from build123d import *

# Parameters (mm, degrees)
SKETCH1_R           = 9.175
SKETCH1_R_2         = 5.6
BOSS_EXTRUDE1_DEPTH = 1.25
CHAMFER1_SIZE       = 0.5
CUT_EXTRUDE1_REACH  = 4.5
CHAMFER2_SIZE       = 0.5


with BuildPart() as part:
    # Sketch1 → Boss-Extrude1 (new body, symmetric)
    with BuildSketch(Plane(origin=(0, 0, 0), x_dir=(1, 0, 0), z_dir=(0, 1, 0))):
        Circle(SKETCH1_R)
        Circle(SKETCH1_R_2, mode=Mode.SUBTRACT)
    extrude(amount=BOSS_EXTRUDE1_DEPTH, both=True)

    # Chamfer1
    chamfer1_edges = [part.edges().sort_by_distance(p)[0] for p in [
        (-9.175, -1.25, 0),
        (-9.175, 1.25, 0),
    ]]
    chamfer(chamfer1_edges, length=CHAMFER1_SIZE)

    # Sketch2 → Cut-Extrude1 (cut, up to next)
    with BuildSketch(Plane(origin=(0, 1.25, 0), x_dir=(1, 0, 0), z_dir=(0, 1, 0)), mode=Mode.PRIVATE) as cut_extrude1_sk1:
        with BuildLine():
            ThreePointArc((-8, 3.354940387), (-8.675, 0), (-8, -3.354940387))
            Line((-8, -3.354940387), (-8, 3.354940387))
        make_face()
    cut_extrude1_tool1 = extrude(cut_extrude1_sk1.sketch, amount=-CUT_EXTRUDE1_REACH, mode=Mode.PRIVATE) & part.part
    add(cut_extrude1_tool1.solids().sort_by_distance((-8.270921, 1.25, 0))[0], mode=Mode.SUBTRACT)
    # Sketch2 → Cut-Extrude1 (cut, up to next)
    with BuildSketch(Plane(origin=(0, 1.25, 0), x_dir=(1, 0, 0), z_dir=(0, 1, 0)), mode=Mode.PRIVATE) as cut_extrude1_sk2:
        with BuildLine():
            ThreePointArc((-8, 4.492285053), (-9.175, 0), (-8, -4.492285053))
            Line((-8, -4.492285053), (-8, -3.354940387))
            ThreePointArc((-8, -3.354940387), (-8.675, 0), (-8, 3.354940387))
            Line((-8, 3.354940387), (-8, 4.492285053))
        make_face()
    cut_extrude1_tool2 = extrude(cut_extrude1_sk2.sketch, amount=-CUT_EXTRUDE1_REACH, mode=Mode.PRIVATE) & part.part
    add(cut_extrude1_tool2.solids().sort_by_distance((-9.084389, 1.25, 0))[0], mode=Mode.SUBTRACT)
    # Sketch2 → Cut-Extrude1 (cut, up to next)
    with BuildSketch(Plane(origin=(0, 1.25, 0), x_dir=(1, 0, 0), z_dir=(0, 1, 0)), mode=Mode.PRIVATE) as cut_extrude1_sk3:
        with BuildLine():
            ThreePointArc((-0.109567023, 9.174345757), (-4.5875, 7.94578308), (-7.890432977, 4.682060704))
            Line((-7.890432977, 4.682060704), (-6.905463603, 5.250733037))
            ThreePointArc((-6.905463603, 5.250733037), (-4.3375, 7.512770378), (-1.094536397, 8.605673424))
            Line((-1.094536397, 8.605673424), (-0.109567023, 9.174345757))
        make_face()
    cut_extrude1_tool3 = extrude(cut_extrude1_sk3.sketch, amount=-CUT_EXTRUDE1_REACH, mode=Mode.PRIVATE) & part.part
    add(cut_extrude1_tool3.solids().sort_by_distance((-4.382423, 1.25, -7.590579))[0], mode=Mode.SUBTRACT)
    # Sketch2 → Cut-Extrude1 (cut, up to next)
    with BuildSketch(Plane(origin=(0, 1.25, 0), x_dir=(1, 0, 0), z_dir=(0, 1, 0)), mode=Mode.PRIVATE) as cut_extrude1_sk4:
        with BuildLine():
            ThreePointArc((-1.094536397, 8.605673424), (-4.3375, 7.512770378), (-6.905463603, 5.250733037))
            Line((-6.905463603, 5.250733037), (-1.094536397, 8.605673424))
        make_face()
    cut_extrude1_tool4 = extrude(cut_extrude1_sk4.sketch, amount=-CUT_EXTRUDE1_REACH, mode=Mode.PRIVATE) & part.part
    add(cut_extrude1_tool4.solids().sort_by_distance((-4.135461, 1.25, -7.162828))[0], mode=Mode.SUBTRACT)
    # Sketch2 → Cut-Extrude1 (cut, up to next)
    with BuildSketch(Plane(origin=(0, 1.25, 0), x_dir=(1, 0, 0), z_dir=(0, 1, 0)), mode=Mode.PRIVATE) as cut_extrude1_sk5:
        with BuildLine():
            ThreePointArc((1.094536397, 8.605673424), (4.3375, 7.512770378), (6.905463603, 5.250733037))
            Line((6.905463603, 5.250733037), (7.890432977, 4.682060704))
            ThreePointArc((7.890432977, 4.682060704), (4.5875, 7.94578308), (0.109567023, 9.174345757))
            Line((0.109567023, 9.174345757), (1.094536397, 8.605673424))
        make_face()
    cut_extrude1_tool5 = extrude(cut_extrude1_sk5.sketch, amount=-CUT_EXTRUDE1_REACH, mode=Mode.PRIVATE) & part.part
    add(cut_extrude1_tool5.solids().sort_by_distance((7.442871, 1.25, -5.044206))[0], mode=Mode.SUBTRACT)
    # Sketch2 → Cut-Extrude1 (cut, up to next)
    with BuildSketch(Plane(origin=(0, 1.25, 0), x_dir=(1, 0, 0), z_dir=(0, 1, 0)), mode=Mode.PRIVATE) as cut_extrude1_sk6:
        with BuildLine():
            Line((1.094536397, 8.605673424), (6.905463603, 5.250733037))
            ThreePointArc((6.905463603, 5.250733037), (4.3375, 7.512770378), (1.094536397, 8.605673424))
        make_face()
    cut_extrude1_tool6 = extrude(cut_extrude1_sk6.sketch, amount=-CUT_EXTRUDE1_REACH, mode=Mode.PRIVATE) & part.part
    add(cut_extrude1_tool6.solids().sort_by_distance((4.135461, 1.25, -7.162828))[0], mode=Mode.SUBTRACT)
    # Sketch2 → Cut-Extrude1 (cut, up to next)
    with BuildSketch(Plane(origin=(0, 1.25, 0), x_dir=(1, 0, 0), z_dir=(0, 1, 0)), mode=Mode.PRIVATE) as cut_extrude1_sk7:
        with BuildLine():
            Line((8, -3.354940387), (8, -4.492285053))
            ThreePointArc((8, -4.492285053), (8.876390736, -2.321704654), (9.175, 0))
            ThreePointArc((9.175, 0), (8.876390736, 2.321704654), (8, 4.492285053))
            Line((8, 4.492285053), (8, 3.354940387))
            ThreePointArc((8, 3.354940387), (8.504575974, 1.711085182), (8.675, 0))
            ThreePointArc((8.675, 0), (8.504575974, -1.711085182), (8, -3.354940387))
        make_face()
    cut_extrude1_tool7 = extrude(cut_extrude1_sk7.sketch, amount=-CUT_EXTRUDE1_REACH, mode=Mode.PRIVATE) & part.part
    add(cut_extrude1_tool7.solids().sort_by_distance((8.090611, 1.25, 3.923613))[0], mode=Mode.SUBTRACT)
    # Sketch2 → Cut-Extrude1 (cut, up to next)
    with BuildSketch(Plane(origin=(0, 1.25, 0), x_dir=(1, 0, 0), z_dir=(0, 1, 0)), mode=Mode.PRIVATE) as cut_extrude1_sk8:
        with BuildLine():
            Line((8, 3.354940387), (8, -3.354940387))
            ThreePointArc((8, -3.354940387), (8.504575974, -1.711085182), (8.675, 0))
            ThreePointArc((8.675, 0), (8.504575974, 1.711085182), (8, 3.354940387))
        make_face()
    cut_extrude1_tool8 = extrude(cut_extrude1_sk8.sketch, amount=-CUT_EXTRUDE1_REACH, mode=Mode.PRIVATE) & part.part
    add(cut_extrude1_tool8.solids().sort_by_distance((8.270921, 1.25, 0))[0], mode=Mode.SUBTRACT)
    # Sketch2 → Cut-Extrude1 (cut, up to next)
    with BuildSketch(Plane(origin=(0, 1.25, 0), x_dir=(1, 0, 0), z_dir=(0, 1, 0)), mode=Mode.PRIVATE) as cut_extrude1_sk9:
        with BuildLine():
            Line((1.094536397, -8.605673424), (0.109567023, -9.174345757))
            ThreePointArc((0.109567023, -9.174345757), (4.5875, -7.94578308), (7.890432977, -4.682060704))
            Line((7.890432977, -4.682060704), (6.905463603, -5.250733037))
            ThreePointArc((6.905463603, -5.250733037), (4.3375, -7.512770378), (1.094536397, -8.605673424))
        make_face()
    cut_extrude1_tool9 = extrude(cut_extrude1_sk9.sketch, amount=-CUT_EXTRUDE1_REACH, mode=Mode.PRIVATE) & part.part
    add(cut_extrude1_tool9.solids().sort_by_distance((4.382423, 1.25, 7.590579))[0], mode=Mode.SUBTRACT)
    # Sketch2 → Cut-Extrude1 (cut, up to next)
    with BuildSketch(Plane(origin=(0, 1.25, 0), x_dir=(1, 0, 0), z_dir=(0, 1, 0)), mode=Mode.PRIVATE) as cut_extrude1_sk10:
        with BuildLine():
            Line((6.905463603, -5.250733037), (1.094536397, -8.605673424))
            ThreePointArc((1.094536397, -8.605673424), (4.3375, -7.512770378), (6.905463603, -5.250733037))
        make_face()
    cut_extrude1_tool10 = extrude(cut_extrude1_sk10.sketch, amount=-CUT_EXTRUDE1_REACH, mode=Mode.PRIVATE) & part.part
    add(cut_extrude1_tool10.solids().sort_by_distance((4.135461, 1.25, 7.162828))[0], mode=Mode.SUBTRACT)
    # Sketch2 → Cut-Extrude1 (cut, up to next)
    with BuildSketch(Plane(origin=(0, 1.25, 0), x_dir=(1, 0, 0), z_dir=(0, 1, 0)), mode=Mode.PRIVATE) as cut_extrude1_sk11:
        with BuildLine():
            ThreePointArc((-6.905463603, -5.250733037), (-4.3375, -7.512770378), (-1.094536397, -8.605673424))
            Line((-1.094536397, -8.605673424), (-6.905463603, -5.250733037))
        make_face()
    cut_extrude1_tool11 = extrude(cut_extrude1_sk11.sketch, amount=-CUT_EXTRUDE1_REACH, mode=Mode.PRIVATE) & part.part
    add(cut_extrude1_tool11.solids().sort_by_distance((-4.135461, 1.25, 7.162828))[0], mode=Mode.SUBTRACT)
    # Sketch2 → Cut-Extrude1 (cut, up to next)
    with BuildSketch(Plane(origin=(0, 1.25, 0), x_dir=(1, 0, 0), z_dir=(0, 1, 0)), mode=Mode.PRIVATE) as cut_extrude1_sk12:
        with BuildLine():
            ThreePointArc((-7.890432977, -4.682060704), (-4.5875, -7.94578308), (-0.109567023, -9.174345757))
            Line((-0.109567023, -9.174345757), (-1.094536397, -8.605673424))
            ThreePointArc((-1.094536397, -8.605673424), (-4.3375, -7.512770378), (-6.905463603, -5.250733037))
            Line((-6.905463603, -5.250733037), (-7.890432977, -4.682060704))
        make_face()
    cut_extrude1_tool12 = extrude(cut_extrude1_sk12.sketch, amount=-CUT_EXTRUDE1_REACH, mode=Mode.PRIVATE) & part.part
    add(cut_extrude1_tool12.solids().sort_by_distance((-7.442871, 1.25, 5.044206))[0], mode=Mode.SUBTRACT)

    # Chamfer2
    chamfer2_edges = [part.edges().sort_by_distance(p)[0] for p in [
        (-5.6, -1.25, 0),
        (-5.6, 1.25, 0),
    ]]
    chamfer(chamfer2_edges, length=CHAMFER2_SIZE)


solid = part.part
Work out the finished part from the listing and answer in its coordinate system (mm). Coordinates: 2 decimals unless noted, no trailing zeros. Write each loop counter-clockwise with the first axis right and the second up, starting at its lowest first coordinate (ties: lowest second). Pieces come first, ordered by that corner, then holes. Notation, with made-up numbers: M -3,13 L 30,13 A22 cw 30,34 Z; hole C 87.25,45 d11. An arc over 180 degrees is marked long. Use one line per item in the form item = value. Start each with the question number.
1. Each of these flat-tipped pins is pushed along its axis until it touches: P1, Ø1.5, axis at y = 0, z = -5.5, coming from the +X side; P2, Ø1.5, axis at x = 0.5, z = -5, coming from the +Y side; P3, Ø6, axis at x = -4, z = 0, coming from the -Y side. Where does it stop, or does it pass through?
2. The part is cut by section A-A (y = -0.4). Give the vertices of the cut face in (x, z) (3 decimals), plus the area to 3 significant figures.
3. Straight lines are drawn through the part: probe 1 along X at (y, z) = (0.1, 0); probe 2 along Z at (x, y) = (0, 0.4) (3 decimals); probe 3 along X at (y, z) = (-0.45, 3.5). For each, find the intervals that lie inside material, in ascending order. Write a range as from..to.
4. The mould has two halves that part along Z. Classify faces 1 (the face through (-8, 0, 0)), 2 (the face through (-5.595, -0.01, -0.246)), 3 (the face through (7.67, -1.06, 4.45)): released by +Z, released by -Z, zero draft, split by the parting line, or undercut.
5. The part is cut by section B-B (z = 0). Give the vertices of the cut face in (x, y).
6. The part is cut by section C-C (z = -7.5). Give the vertices of the cut face in (x, y).
Evaluation:
q1.P1 = 7.77
q1.P2 = 0.92
q1.P3 = -1.25
q2.outline = M -8,-4.492 A9.175 ccw -7.89,-4.682 L -0.11,-9.174 A9.175 ccw 0.11,-9.174 L 7.89,-4.682 A9.175 ccw 8,-4.492 L 8,4.492 A9.175 ccw 7.89,4.682 L 0.11,9.174 A9.175 ccw -0.11,9.174 L -7.89,4.682 A9.175 ccw -8,4.492 Z; hole C 0,0 d11.2
q2.area = 123 mm^2
q3.probe_1 = -8..-5.6, 5.6..8
q3.probe_2 = -9.175..-5.6, 5.6..9.175
q3.probe_3 = -8..-4.37, 4.37..8
q4.face_1 = zero draft
q4.face_2 = undercut
q4.face_3 = released by +Z
q5.outline = M -8,-1.25 L -6.1,-1.25 L -5.6,-0.75 L -5.6,0.75 L -6.1,1.25 L -8,1.25 Z; M 5.6,-0.75 L 6.1,-1.25 L 8,-1.25 L 8,1.25 L 6.1,1.25 L 5.6,0.75 Z
q6.outline = M -3.01,-1.25 L 3.01,-1.25 L 3.01,1.25 L -3.01,1.25 Z
